Design review of the part built by this model. Coordinates are the model's own, in mm. A direction names the side the tool comes from. Coordinates: 2 decimals unless noted, no trailing zeros. Write each loop counter-clockwise with the first axis right and the second up, starting at its lowest first coordinate (ties: lowest second). Pieces come first, ordered by that corner, then holes.
Q1. Add section A-A, the plane y = 0. Give the number of separate pieces and of enclosed holes in the cut face, plus the area to 3 significant figures.
Q2. The part is to be moulded in two halves that separate along Z. For faces 1 (the face through (-0.85, -3.827, 0.76)), 2 (the face through (-0.65, 8.84, 1.98)), 3 (the face through (0, -9, 6.124)), say which applies: +Z half, -Z half, draft (parallel to the pull), parting line (faces both ways), or undercut.
Q3. Clearance check with flat-ended pins moving along their axes: pin 1 Ø1.6 at (y, z) = (-8, 8) entering from -X; pin 2 Ø2 at (x, z) = (5.5, 7.5) entering from -Y; pin 3 Ø0.8 at (x, z) = (7, 6) entering from -Y. State where each tip first meets the part, or that it passes through.
Q4. Add section C-C, the plane z = 5.75. Give the boundary of the cut face in (x, y), plus the area to 3 significant figures.
Q5. Machinability: for faces 4 (the face through (3.937, -8, 7)), 5 (the face through (-2.17, -9.76, 4.44)), 6 (the face through (-8.3, 1.7, 7.5)), 7 (the face through (-7, -5.59, 4)), which of the approach directions +Z, -Z, +X, -X, +Y, -Y give a long, thin tool a straight path to every point of the face, cutting with its end or side? Answer none if there is none.
Q6. Add section D-D, the plane y = 7.25. Give the boundary of the cut face in (x, z), plus the area to 3 significant figures.
Q7. To check wall thickness, follow probe 1 along Z at (x, y) = (-7.25, -4.25); probe 2 along Z at (x, y) = (8, 4.25); probe 3 along X at (y, z) = (0, 5). State the ranges of each line that lie inside material, in increasing order.
Q8. Add section B-B, the plane x = 0. Give the boundary of the cut face in (y, z), plus the area to 3 significant figures.
from build123d import *

# Parameters (mm, degrees)
F0_R      = 10
F1_DEPTH  = 9
F2_R      = 9
F3_DEPTH  = 1.5
F4_R      = 8.25
F5_DEPTH  = 6
F6_R      = 3.92
F7_DEPTH  = 1.501
F8_R      = 3
F9_DEPTH  = 10.001
F10_W     = 8.018549
F10_H     = 2.886699
F11_DEPTH = 25
F12_W     = 11.538846
F12_H     = 1.004787
F13_DEPTH = 25


with BuildPart() as f1:
    # F0 (on Top) → F1 (new body)
    with BuildSketch(Plane.XY):
        Circle(F0_R)
    extrude(amount=F1_DEPTH)

    # F2 (on face) → F3 (cut)
    with BuildSketch(Plane.XY.offset(9)):
        Circle(F2_R)
    extrude(amount=-F3_DEPTH, mode=Mode.SUBTRACT)

    # F4 (on face) → F5 (cut)
    with BuildSketch(Plane.XY.offset(7.5)):
        Circle(F4_R)
    extrude(amount=-F5_DEPTH, mode=Mode.SUBTRACT)

    # F6 (on face) → F7 (cut, through all)
    with BuildSketch(Plane.XY.offset(1.5)):
        Circle(F6_R)
    extrude(amount=-F7_DEPTH, mode=Mode.SUBTRACT)

    # F8 (on Front) → F9 (cut, through all)
    with BuildSketch(Plane.XZ):
        with Locations((0, 4.907787)):
            Circle(F8_R)
    extrude(amount=-F9_DEPTH, mode=Mode.SUBTRACT)

    # F10 (on Front) → F11 (cut)
    with BuildSketch(Plane.XZ):
        with Locations((-0.07208, 7.567474)):
            Rectangle(F10_W, F10_H)
    extrude(amount=F11_DEPTH, mode=Mode.SUBTRACT)

    # F12 (on Right) → F13 (cut, symmetric)
    with BuildSketch(Plane.YZ):
        with Locations((0.171022, 5.98548)):
            Rectangle(F12_W, F12_H)
        with Locations((0.179522, 4.236611)):
            Rectangle(F12_W, F12_H)
    extrude(amount=F13_DEPTH, both=True, mode=Mode.SUBTRACT)


solid = f1.part
Here are the results:
1. separate pieces: 6
1. enclosed holes: 0
1. area: 35.2 mm2
2. face 1: draft
2. face 2: undercut
2. face 3: +Z half
3. pin 1: stops at x = -6.94
3. pin 2: stops at y = -8.93
3. pin 3: stops at y = -7.51
4. outline: (-8.29, -5.6) arc R10 ccw to (8.29, -5.6) - (6.06, -5.6) arc R8.25 cw to (-6.06, -5.6) - close; (-8.04, 5.94) - (-5.72, 5.94) arc R8.25 cw to (-2.88, 7.73) - (-2.88, 9.58) arc R10 ccw to start; (2.88, 7.73) arc R8.25 cw to (5.72, 5.94) - (8.04, 5.94) arc R10 ccw to (2.88, 9.58) - close
4. area: 46.3 mm2
5. face 4: +Z, -Y
5. face 5: +Z, -Z
5. face 6: +Z
5. face 7: +X, -X
6. outline: (-6.89, 0) - (6.89, 0) - (6.89, 9) - (5.33, 9) - (5.33, 7.5) - (3.94, 7.5) - (3.94, 1.5) - (-3.94, 1.5) - (-3.94, 7.5) - (-5.33, 7.5) - (-5.33, 9) - (-6.89, 9) - close
6. area: 60.7 mm2
7. probe 1: z = 0 to 3.73, 4.74 to 5.48, 6.49 to 7.5
7. probe 2: z = 0 to 3.73, 4.74 to 5.48, 6.49 to 9
7. probe 3: x = -10 to -8.25, 8.25 to 10
8. outline: (-10, 0) - (-3.92, 0) - (-3.92, 1.5) - (-8.25, 1.5) - (-8.25, 6.12) - (-10, 6.12) - close; (3.92, 0) - (10, 0) - (10, 1.91) - (8.25, 1.91) - (8.25, 1.5) - (3.92, 1.5) - close; (9, 7.91) - (10, 7.91) - (10, 9) - (9, 9) - close
8. area: 28.1 mm2
